Check sheet for the modelled part. Datum: model origin and axes. Units: mm. Round coordinates to 2 decimals unless told otherwise and drop trailing zeros. Loops run counter-clockwise (first coordinate to the right, second up) from the corner with the lowest first, then second, coordinate; pieces in that order, holes last. Notation, with made-up numbers: (16.25, 76.25) - (65.25, 76.25) arc R24 cw to (65.25, 111.25) - close; hole circle Ø6 at (-34, 6.5). An arc over 180 degrees is marked (long way). Answer in a Markdown table with one row per item. Add a question column.
(1) Thickness scan on line 1 along Y through (x, z) = (-2, 8.25); line 2 along Y through (x, z) = (2, 9); line 3 along Y through (x, z) = (0, 16). Record the ranges inside material, lowest first.
(2) Cross-section at A-A on z = 14.25. Enter the section's corners in (x, y).
(3) Gauge pin test, flat ends, axial feed: pin 1 (1 mm diameter, centred on x = 0.5, y = -0.5, fed in from +Z); pin 2 (2 mm diameter, centred on y = -0.5, z = 7.5, fed in from +X). Record the tip position at first contact, or that the pin passes through.
(4) Cross-section at D-D on y = -5. Enter the section's corners in (x, z).
(5) Cross-section at B-B on z = 5.5. Enter the section's corners in (x, y), then the cut area to 3 significant figures.
(6) Cross-section at C-C on x = 9. Enter the section's corners in (y, z), then the cut area to 3 significant figures.
from build123d import *

# Parameters (mm, degrees)
F0_W     = 30
F0_H     = 21
F0_R     = 3
F1_DEPTH = 17
F3_DEPTH = 35
F4_DEPTH = 10
F5_R     = 1
F6_R     = 2


with BuildPart() as f1:
    # F0 (on Top) → F1 (new body)
    with BuildSketch(Plane.XY):
        Rectangle(F0_W, F0_H)
        Circle(F0_R, mode=Mode.SUBTRACT)
    extrude(amount=F1_DEPTH)

    # F2 (on face) → F3 (cut)
    with BuildSketch(Plane(origin=(-15, 0, 0), x_dir=(0, -1, 0), z_dir=(-1, 0, 0))):
        with BuildLine():
            ThreePointArc((-5.5756953559, 17), (-3.1140357378, 3.8940927926), (8, 11.2631348893))
            ThreePointArc((8, 11.2631348893), (7.3690420967, 14.3771706271), (5.5756953559, 17))
            Line((5.5756953559, 17), (-5.5756953559, 17))
        make_face()
    extrude(amount=-F3_DEPTH, mode=Mode.SUBTRACT)

    # F0 (on Top) → F4 (join)
    with BuildSketch(Plane.XY):
        Circle(F0_R)
    extrude(amount=F4_DEPTH)

    # F5
    f5_edges = [f1.edges().sort_by_distance(p)[0] for p in [
        (0, -10.5, 17),
        (0, 10.5, 17),
        (0, 5.575695, 17),
        (0, -5.575695, 17),
        (0, -10.5, 0),
        (0, 10.5, 0),
        (-15, 10.5, 8.5),
        (15, 10.5, 8.5),
        (15, -10.5, 8.5),
        (-15, -10.5, 8.5),
    ]]
    fillet(f5_edges, radius=F5_R)

    # F6
    f6_edges = [f1.edges().sort_by_distance(p)[0] for p in [
        (-3, 0, 10),
    ]]
    fillet(f6_edges, radius=F6_R)


solid = f1.part
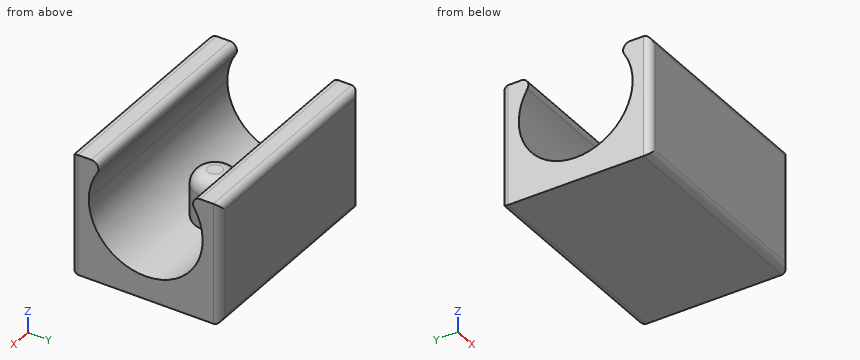
Answers:
| question | item | result |
|---|---|---|
| 1 | line 1 | y = -10.5 to -7.41, -2.21 to 2.21, 7.41 to 10.5 |
| 1 | line 2 | y = -10.5 to -7.67, -1.86 to 1.86, 7.67 to 10.5 |
| 1 | line 3 | y = -10.5 to -6.65, 6.65 to 10.5 |
| 2 | outline | (-15, -9.5) arc R1 ccw to (-14, -10.5) - (14, -10.5) arc R1 ccw to (15, -9.5) - (15, -7.42) - (-15, -7.42) - close; (-15, 7.42) - (15, 7.42) - (15, 9.5) arc R1 ccw to (14, 10.5) - (-14, 10.5) arc R1 ccw to (-15, 9.5) - close |
| 3 | pin 1 | stops at z = 10 |
| 3 | pin 2 | stops at x = 3 |
| 4 | outline | (-15, 0) - (15, 0) - (15, 5.02) - (-15, 5.02) - close |
| 5 | outline | (-15, -9.5) arc R1 ccw to (-14, -10.5) - (14, -10.5) arc R1 ccw to (15, -9.5) - (15, -5.55) - (-15, -5.55) - close; (-15, 5.55) - (15, 5.55) - (15, 9.5) arc R1 ccw to (14, 10.5) - (-14, 10.5) arc R1 ccw to (-15, 9.5) - close; circle Ø6 at (0, 0) |
| 5 | area | 325 mm^2 |
| 6 | outline | (-10.5, 1) arc R1 ccw to (-9.5, 0) - (9.5, 0) arc R1 ccw to (10.5, 1) - (10.5, 16) arc R1 ccw to (9.5, 17) - (7.65, 17) arc R1 ccw to (6.8, 15.47) arc R8 cw (long way) to (-6.8, 15.47) arc R1 ccw to (-7.65, 17) - (-9.5, 17) arc R1 ccw to (-10.5, 16) - close |
| 6 | area | 171 mm^2 |
